Can you work these out from the model? Positions are in its coordinate system, mm. Face numbers are marked on the shaded views. A direction names the side the tool comes from. Coordinates: 2 decimals unless noted, no trailing zeros. Loops run counter-clockwise (first coordinate to the right, second up) from the corner with the lowest first, then second, coordinate; pieces in that order, holes last. Notation, with made-up numbers: (68, -18.5) -> (121, -18.5) arc R14 ccw to (121, -10.5) -> close; hole circle Ø4 at (-5.75, 16). An arc over 180 degrees is marked (long way). Use one line per item in the form item = value. Start each with the question number.
(1) Imagine slicing it at D-D (y = 601). List the corners of the cut face in (x, z) for me.
(2) Imagine slicing it at B-B (x = 175). List the corners of the cut face in (y, z) for me.
(3) I'm going to push flat-ended pins straight in: pin 1 (10 mm diameter, centred on x = 182.5, z = -18.5, fed in from -Y); pin 2 (7.5 mm diameter, centred on y = 597, z = -22, fed in from -X); pin 3 (3 mm diameter, centred on y = 603.46, z = -25.64, fed in from -X); pin 4 (5 mm diameter, centred on y = 603.46, z = -25.64, fed in from +X). Where does each tip first touch, or does it pass through?
(4) I need wall thicknesses on line 1 (X direction, y = 606.75, z = -18.5); line 2 (Z direction, x = 181, y = 604.25); line 3 (Z direction, x = 179.5, y = 593). Which ranges of each line are inside material? Lowest first, please. Write a range as [from, to].
(5) Thinking about a two-plate mould opening in X: for the marked faces 1, 2 and 3, which applies, released by +X, released by -X, zero draft, split by the parting line, or undercut?
(6) On a 3-axis mill with a long thin cutter (end or side, diameter ignored), from which of +Z, -Z, +X, -X, +Y, -Y can I reach the whole of each face in a straight line? I mean the marked faces 4 and 5. Say none if no direction works.
(7) Imagine slicing it at C-C (z = -20). List the corners of the cut face in (x, y) for me, plus the area to 3 significant figures.
(8) Imagine slicing it at A-A (y = 603.25). List the corners of the cut face in (x, z) for me, plus the area to 3 significant figures.
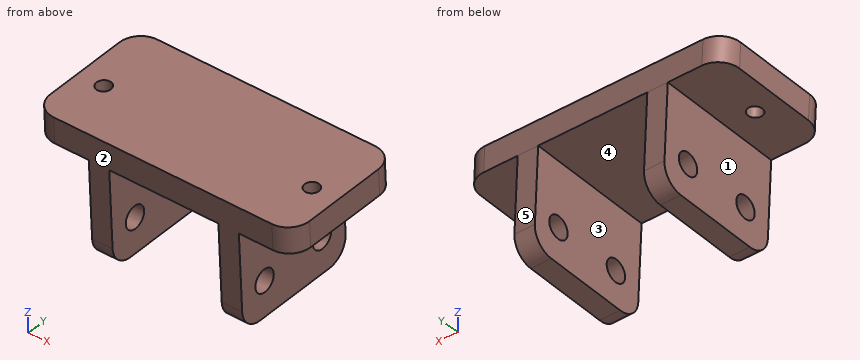
Solid Edge part; units mm, degrees
sketch "Sketch1" plane through (198.5468, 0, 0) normal (1, 0, 0) x (0, 1, 0)
  line L0 (588.9141, -15.3741) -> (589.7381, -31.3529)
  line L1 (589.7381, -31.3529) -> (607.7142, -30.426)
  line L2 (607.7142, -30.426) -> (606.8902, -14.4472)
  line L3 (606.8902, -14.4472) -> (588.9141, -15.3741)
extrude "Protrusion1" add sketch "Sketch1" along normal blind 3
mirror "Mirror1" about plane through (190.5468, 0, 0) normal (1, 0, 0) of "Protrusion1"
sketch "Sketch2" plane through (200.0468, 589.3261, -23.3635) normal (0, -0.9987, -0.0515) x (0, 0.0515, -0.9987)
  line L0 (-9.8549, 9.5) -> (-9.8549, -28.5)
  line L1 (-9.8549, -28.5) -> (-6.1449, -28.5)
  line L2 (-6.1449, -28.5) -> (-6.1449, 9.5)
  line L3 (-6.1449, 9.5) -> (-9.8549, 9.5)
extrude "Protrusion2" add sketch "Sketch2" against normal up to vertex (18 mm away)
fillet "Round_2" radius 3 8 edges at (209.5468, 588.9141, -15.3741) (209.5468, 606.8902, -14.4472) (200.0468, 589.7381, -31.3529) (200.0468, 607.7142, -30.426) (181.0468, 589.7381, -31.3529) (171.5468, 588.9141, -15.3741) (181.0468, 607.7142, -30.426) (171.5468, 606.8902, -14.4472)
sketch "Sketch3" plane through (190.5468, 597.8066, -13.0581) normal (0, -0.0515, 0.9987) x (-1, 0, 0)
  circle A0 centre (-15.25, 1.1575) radius 1.05
  circle A1 centre (15.25, 1.1575) radius 1.05
extrude "Cutout1" cut sketch "Sketch3" against normal up to next
sketch "Sketch4" plane through (201.5468, 598.2866, -23.751) normal (1, 0, 0) x (0, -0.9987, -0.0515)
  circle A0 centre (4.9287, 2.1516) radius 1.6
  circle A1 centre (-5.0713, 2.1516) radius 1.6
extrude "Cutout2" cut sketch "Sketch4" against normal through all
properties material "ABS 40% Infill"
Worked out:
q1.outline = (171.55, -16.61) -> (179.55, -16.61) -> (179.55, -30.77) -> (182.55, -30.77) -> (182.55, -16.61) -> (198.55, -16.61) -> (198.55, -30.77) -> (201.55, -30.77) -> (201.55, -16.61) -> (209.55, -16.61) -> (209.55, -12.89) -> (171.55, -12.89) -> close
q2.outline = (588.82, -13.52) -> (589.01, -17.23) -> (595.84, -16.87) -> (595.64, -13.17) -> close; (597.66, -13.07) -> (597.85, -16.77) -> (606.99, -16.3) -> (606.79, -12.59) -> close
q3.pin_1 = 588.82
q3.pin_2 = 179.55
q3.pin_3 = through
q3.pin_4 = 201.55
q4.line_1 = [179.55, 182.55], [198.55, 201.55]
q4.line_2 = [-30.6, -27.03], [-24.25, -12.73]
q4.line_3 = [-17.02, -13.31]
q5.face_1 = released by -X
q5.face_2 = zero draft
q5.face_3 = undercut
q6.face_4 = -Z, +Y
q6.face_5 = +Z, +X, -X, +Y
q7.outline = (179.55, 589.15) -> (182.55, 589.15) -> (182.55, 607.18) -> (179.55, 607.18) -> close; (198.55, 589.15) -> (201.55, 589.15) -> (201.55, 607.18) -> (198.55, 607.18) -> close
q7.area = 108 mm2
q8.outline = (171.55, -16.49) -> (179.55, -16.49) -> (179.55, -24.05) -> (182.55, -24.05) -> (182.55, -16.49) -> (198.55, -16.49) -> (198.55, -24.05) -> (201.55, -24.05) -> (201.55, -16.49) -> (209.55, -16.49) -> (209.55, -12.78) -> (171.55, -12.78) -> close; (179.55, -30.66) -> (182.55, -30.66) -> (182.55, -27.22) -> (179.55, -27.22) -> close; (198.55, -30.66) -> (201.55, -30.66) -> (201.55, -27.22) -> (198.55, -27.22) -> close
q8.area = 207 mm2
